Geometry check sheet. Reference: the model listing, model coordinates, mm. A direction names the side the tool comes from. Coordinates: 2 decimals unless noted, no trailing zeros. Order: outer loops, then holes, each group sorted by start corner. A loop starts at its lowest first (then second) coordinate and runs counter-clockwise, first axis right, second up. Notation, with made-up numbers: (64.5, 18) - (75.5, 18) arc R25 cw to (75.5, 51) - close; hole circle Ø9 at (76, 62). An arc over 180 degrees is marked (long way). Put each result on its own line as item: value.
from build123d import *

# Parameters (mm, degrees)
SKETCH1_W           = 196.342
SKETCH1_H           = 50.8
BOSS_EXTRUDE1_DEPTH = 3.175
CUT_EXTRUDE1_DEPTH  = 7.62


with BuildPart() as part:
    # Sketch1 → Boss-Extrude1 (new body)
    with BuildSketch(Plane(origin=(0, 0, 0), x_dir=(1, 0, 0), z_dir=(0, 1, 0))):
        with Locations((98.171, 25.4)):
            Rectangle(SKETCH1_W, SKETCH1_H)
    extrude(amount=BOSS_EXTRUDE1_DEPTH)

    # Sketch2 → Cut-Extrude1 (cut)
    with BuildSketch(Plane.XZ):
        Polygon((136.525, -25.7175), (136.525, -36.83), (133.35, -36.83), (133.35, -11.43), (136.525, -11.43), (136.525, -22.5425), (149.225, -22.5425), (149.225, -11.43), (152.4, -11.43), (152.4, -36.83), (149.225, -36.83), (149.225, -25.7175), align=None)
    extrude(amount=-CUT_EXTRUDE1_DEPTH, mode=Mode.SUBTRACT)


solid = part.part
Q1. Section check B-B on z = -18.5. Record the boundary of the cut face in (x, y) (3 decimals), then the cut area to 3 significant figures.
Answer block:
outline: (0, 0) - (133.35, 0) - (133.35, 3.175) - (0, 3.175) - close; (136.525, 0) - (149.225, 0) - (149.225, 3.175) - (136.525, 3.175) - close; (152.4, 0) - (196.342, 0) - (196.342, 3.175) - (152.4, 3.175) - close
area: 603 mm^2
Q2. Access from +Z, -Z, +X, -X, +Y, -Y to the whole of each face (thin tool, end or side, straight path). Record for faces 1 (the flat face through (196.342, 2, -25)), 2 (the flat face through (143, 2, -22.542)).
Answer block:
face 1: +Z, -Z, +X, +Y, -Y
face 2: +Y, -Y
Q3. Thickness scan on L1, parallel to X at y = 2.7, z = -17 (3 decimals); L2, parallel to X at y = 2.2, z = -25; L3, parallel to Z at x = 145, y = 0.5. Record the ranges inside material, lowest first. Write a range as [from, to].
Answer block:
L1: x = [0, 133.35], [136.525, 149.225], [152.4, 196.342]
L2: x = [0, 133.35], [152.4, 196.34]
L3: z = [-50.8, -25.72], [-22.54, 0]
Q4. Draft check along X on faces 3 (the flat face through (149.225, 2, -31)), 4 (the flat face through (97, 3.175, -26)), 5 (the flat face through (0, 2, -25)). Enter one of: pulls with the +X half, pulls with the -X half, needs draft (parallel to the pull), parting line crosses it, or undercut.
Answer block:
face 3: undercut
face 4: needs draft
face 5: pulls with the -X half
